The drawing under review shows one solid part. Ordinate dimensions are in mm from its lowest x, y, z. A direction names the side the tool comes from. Coordinates: 2 decimals unless noted, no trailing zeros. Order: outer loops, then holes, each group sorted by start corner. A loop starts at its lowest first (then second) coordinate and runs counter-clockwise, first axis right, second up.
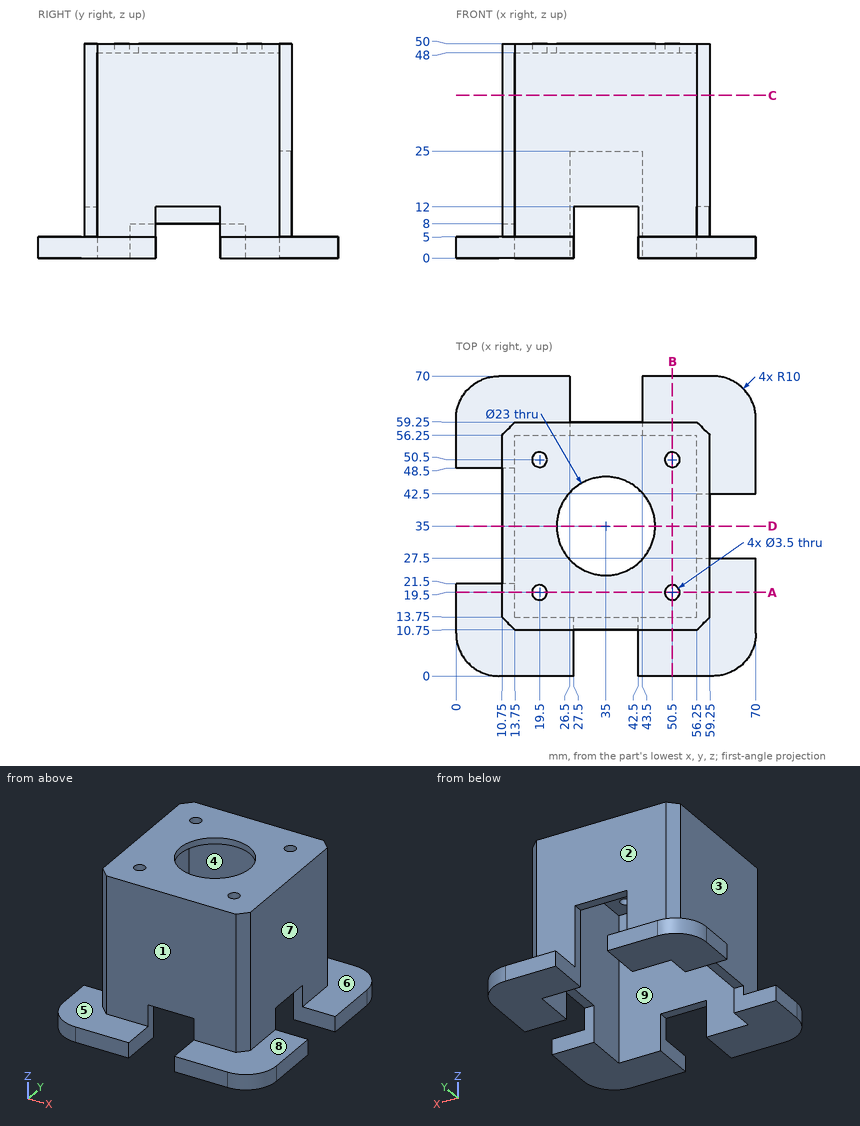
(1) Wall thickness on probe 1 along Y at (x, z) = (19.5, 49.5); probe 2 along Y at (x, z) = (55, 13.5): over which ranges is each line inside the solid? List them lowest first.
A:
probe 1: y = 10.75 to 17.75, 21.25 to 48.75, 52.25 to 59.25
probe 2: y = 10.75 to 13.75, 56.25 to 59.25
(2) We need section D-D, the plane y = 35. Write out the cut boundary in (x, z).
A:
outline: (10.75, 8) - (13.75, 8) - (13.75, 48) - (23.5, 48) - (23.5, 50) - (10.75, 50) - close; (46.5, 48) - (56.25, 48) - (56.25, 12) - (59.25, 12) - (59.25, 50) - (46.5, 50) - close
(3) We need section A-A, the plane y = 19.5. Write out the cut boundary in (x, z), and give its area (4 significant figures).
A:
outline: (0, 0) - (13.75, 0) - (13.75, 48) - (17.75, 48) - (17.75, 50) - (10.75, 50) - (10.75, 5) - (0, 5) - close; (21.25, 48) - (48.75, 48) - (48.75, 50) - (21.25, 50) - close; (52.25, 48) - (56.25, 48) - (56.25, 0) - (70, 0) - (70, 5) - (59.25, 5) - (59.25, 50) - (52.25, 50) - close
area: 478.5 mm2
(4) For pin 1 Ø13 at (x, z) = (32.5, 27.5) entering from +Y; pin 2 Ø0.9 at (x, y) = (11.5, 38.5) entering from -Z; pin 3 Ø2 at (x, z) = (39, 24.5) entering from -Y; pin 4 Ø2 at (x, y) = (19.5, 50.5) entering from +Z, all flat-tipped, find the tip position at first contact; note any pin that passes through.
A:
pin 1: stops at y = 59.25
pin 2: stops at z = 8
pin 3: stops at y = 10.75
pin 4: passes through
(5) Machinability: for the marked faces 5, 6, 7, 8 and 9, which of the approach directions +Z, -Z, +X, -X, +Y, -Y give a long, thin tool a straight path to every point of the face, cutting with its end or side? Answer none if there is none.
A:
face 5: +Z, -X, -Y
face 6: +Z, +X, +Y
face 7: +Z, +X, +Y, -Y
face 8: +Z, +X, -Y
face 9: -Z
(6) We need section C-C, the plane z = 38. Write out the cut boundary in (x, y), and give its area (3 significant figures).
A:
outline: (10.75, 13.75) - (13.75, 10.75) - (56.25, 10.75) - (59.25, 13.75) - (59.25, 56.25) - (56.25, 59.25) - (13.75, 59.25) - (10.75, 56.25) - close; hole (13.75, 13.75) - (56.25, 13.75) - (56.25, 56.25) - (13.75, 56.25) - close
area: 528 mm2
(7) Draft analysis for pull direction Y (two halves, no side actions). For the marked faces 1, 2, 3 and 4, state which applies: released by +Y, released by -Y, zero draft, split by the parting line, or undercut.
A:
face 1: released by -Y
face 2: released by +Y
face 3: zero draft
face 4: undercut
